from build123d import *

# Parameters (mm, degrees)
SKETCH2_R           = 12.5
BOSS_EXTRUDE1_DEPTH = 13
SKETCH3_R           = 2.45
BOSS_EXTRUDE2_DEPTH = 26
SKETCH4_R           = 12.9
BOSS_EXTRUDE3_DEPTH = 13
SKETCH5_R           = 2.625
BOSS_EXTRUDE4_DEPTH = 26
SKETCH6_R           = 4.9
BOSS_EXTRUDE5_DEPTH = 15
SKETCH7_R           = 13.125
BOSS_EXTRUDE6_DEPTH = 13
SKETCH8_R           = 13.125
SKETCH8_R_2         = 12.95
CUT_EXTRUDE1_DEPTH  = 44.191796096


with BuildPart() as part:
    # Sketch2 → Boss-Extrude1 (new body)
    with BuildSketch(Plane.XY):
        with Locations(Location((0, 0, 0), (0, 0, 180))):
            Circle(SKETCH2_R)
    extrude(amount=BOSS_EXTRUDE1_DEPTH)

    # Sketch3 → Boss-Extrude2 (add)
    with BuildSketch(Plane.XY.offset(13)):
        with Locations(Location((0, 0, 0), (0, 0, 180))):
            Circle(SKETCH3_R)
    extrude(amount=BOSS_EXTRUDE2_DEPTH)

    # Sketch4 → Boss-Extrude3 (add)
    with BuildSketch(Plane(origin=(0, 0, 0), x_dir=(-1, 0, 0), z_dir=(0, 0, -1))):
        Circle(SKETCH4_R)
    extrude(amount=-BOSS_EXTRUDE3_DEPTH)

    # Sketch5 → Boss-Extrude4 (add)
    with BuildSketch(Plane.XY.offset(39)):
        Circle(SKETCH5_R)
    extrude(amount=-BOSS_EXTRUDE4_DEPTH)

    # Sketch6 → Boss-Extrude5 (add)
    with BuildSketch(Plane.XY.offset(13)):
        Circle(SKETCH6_R)
    extrude(amount=BOSS_EXTRUDE5_DEPTH)

    # Sketch7 → Boss-Extrude6 (add)
    with BuildSketch(Plane(origin=(0, 0, 0), x_dir=(-1, 0, 0), z_dir=(0, 0, -1))):
        Circle(SKETCH7_R)
    extrude(amount=-BOSS_EXTRUDE6_DEPTH)

    # Sketch8 → Cut-Extrude1 (cut, through all)
    with BuildSketch(Plane(origin=(0, 0, 0), x_dir=(-1, 0, 0), z_dir=(0, 0, -1))):
        Circle(SKETCH8_R)
        Circle(SKETCH8_R_2, mode=Mode.SUBTRACT)
    extrude(amount=-CUT_EXTRUDE1_DEPTH, mode=Mode.SUBTRACT)


solid = part.part
Read the model definition and answer for the solid it produces. Units are mm, in the model's axes. A direction names the side the tool comes from. Coordinates: 2 decimals unless noted, no trailing zeros. Write each loop counter-clockwise with the first axis right and the second up, starting at its lowest first coordinate (ties: lowest second). Pieces come first, ordered by that corner, then holes. Notation, with made-up numbers: M 1,76 L 39,76 A20 ccw 39,81 Z; hole C -33.5,-4.75 d8. An arc over 180 degrees is marked long. Use a Markdown table: item, result.
Q1. Which of the six approach directions +Z, -Z, +X, -X, +Y, -Y give full straight-line access (tool end or side, diameter ignored) to faces 1 (the face through (2, -2, 28)), 2 (the face through (0, 0, 39))?
Answer block:
| item | result |
|---|---|
| face 1 | +Z |
| face 2 | +Z, +X, -X, +Y, -Y |
Q2. The part is cut by section A-A, the plane y = 0. Write down the section's boundary in (x, z) (3 decimals), then the cut area to 3 significant figures.
Answer block:
| item | result |
|---|---|
| outline | M -12.95,0 L 12.95,0 L 12.95,13 L 4.9,13 L 4.9,28 L 2.625,28 L 2.625,39 L -2.625,39 L -2.625,28 L -4.9,28 L -4.9,13 L -12.95,13 Z |
| area | 541 mm2 |
Q3. Each of these flat-tipped pins is pushed along its axis until it touches: pin 1 Ø4 at (x, y) = (6.5, 10) entering from +Z; pin 2 Ø5 at (x, y) = (-5, 4.5) entering from +Z; pin 3 Ø2 at (y, z) = (4, 32.5) entering from +X. Where does it stop, or does it pass through?
Answer block:
| item | result |
|---|---|
| pin 1 | stops at z = 13 |
| pin 2 | stops at z = 28 |
| pin 3 | passes through |
Q4. The part is cut by section D-D, the plane x = 3.25. Write down the section's boundary in (y, z).
Answer block:
| item | result |
|---|---|
| outline | M -12.54,0 L 12.54,0 L 12.54,13 L 3.67,13 L 3.67,28 L -3.67,28 L -3.67,13 L -12.54,13 Z |
Q5. Straight lines are drawn through the part: L1, parallel to Z at x = 0, y = -10.75; L2, parallel to Y at x = 10.25, z = 4; L3, parallel to Y at x = -0.25, z = 15.5. For each, find the intervals that lie inside material, in ascending order. Write a range as [from, to].
Answer block:
| item | result |
|---|---|
| L1 | z = [0, 13] |
| L2 | y = [-7.91, 7.91] |
| L3 | y = [-4.89, 4.89] |
Q6. The part is cut by section C-C, the plane z = 6. Write down the section's boundary in (x, y).
Answer block:
| item | result |
|---|---|
| outline | C 0,0 d25.9 |
